from build123d import *

# Parameters (mm, degrees)
BOSS_EXTRUDE1_DEPTH = 133.35
SKETCH2_R           = 1.2
SKETCH2_R_2         = 19.75
CUT_EXTRUDE1_DEPTH  = 187.593999065
SKETCH3_W           = 133.35
SKETCH3_H           = 3.175
BOSS_EXTRUDE2_DEPTH = 3.175
FILLET1_R           = 3.175
SKETCH5_R           = 15
CUT_EXTRUDE2_DEPTH  = 189.467318942
SKETCH6_R           = 6
SKETCH6_R_2         = 5.999988
CUT_EXTRUDE3_DEPTH  = 189.467318942


with BuildPart() as part:
    # Sketch1 → Boss-Extrude1 (new body)
    with BuildSketch(Plane.XY):
        Polygon((110.49, -69.425000088), (0, 0), (0, 3.175), (110.49, -66.250000088), align=None)
    extrude(amount=BOSS_EXTRUDE1_DEPTH)

    # Sketch2 → Cut-Extrude1 (cut, through all)
    with BuildSketch(Plane(origin=(1.430283892, 2.276299128, 0), x_dir=(0.8467258159330607, -0.5320295035357462, 0), z_dir=(0.5320295035357462, 0.8467258159330607, 0))):
        with Locations(Location((26.260806326, -83.175, 0), (0, 0, 180))):
            Circle(SKETCH2_R)
        with Locations(Location((42.760806326, -66.675, 0), (0, 0, 180))):
            Circle(SKETCH2_R_2)
        with Locations(Location((59.260806326, -83.175, 0), (0, 0, 180))):
            Circle(SKETCH2_R)
        with Locations(Location((26.260806326, -50.175, 0), (0, 0, 180))):
            Circle(SKETCH2_R)
        with Locations(Location((59.260806326, -50.175, 0), (0, 0, 180))):
            Circle(SKETCH2_R)
    extrude(amount=-CUT_EXTRUDE1_DEPTH, mode=Mode.SUBTRACT)

    # Sketch3 → Boss-Extrude2 (add)
    with BuildSketch(Plane(origin=(110.49, 0, 0), x_dir=(0, 0, -1), z_dir=(1, 0, 0))):
        with Locations((-66.675, -67.837500088)):
            Rectangle(SKETCH3_W, SKETCH3_H)
    extrude(amount=BOSS_EXTRUDE2_DEPTH)

    # Fillet1
    fillet1_edges = [part.edges().sort_by_distance(p)[0] for p in [
        (113.665, -66.250000088, 66.675),
    ]]
    fillet(fillet1_edges, radius=FILLET1_R - 0.0001)  # a hair under: the kernel refuses the full size

    # Sketch5 → Cut-Extrude2 (cut, through all)
    with BuildSketch(Plane(origin=(1.430283892, 2.276299128, 0), x_dir=(0.8467258159330606, -0.5320295035357464, 0), z_dir=(0.5320295035357464, 0.8467258159330606, 0))):
        with Locations(Location((20.851690059, -111.125, 0), (0, 0, 180))):
            Circle(SKETCH5_R)
        with Locations(Location((20.851690059, -22.225, 0), (0, 0, 180))):
            Circle(SKETCH5_R)
    extrude(amount=-CUT_EXTRUDE2_DEPTH, mode=Mode.SUBTRACT)

    # Sketch6 → Cut-Extrude3 (cut, through all)
    with BuildSketch(Plane(origin=(1.430283892, 2.276299128, 0), x_dir=(0.8467258159330606, -0.5320295035357464, 0), z_dir=(0.5320295035357464, 0.8467258159330606, 0))):
        with Locations(Location((87.210806326, -46.355, 0), (0, 0, 180))):
            Circle(SKETCH6_R)
        with Locations(Location((87.210806326, -26.035, 0), (0, 0, 180))):
            Circle(SKETCH6_R)
        with Locations(Location((87.210806326, -86.995, 0), (0, 0, 180))):
            Circle(SKETCH6_R)
        with Locations(Location((87.210806326, -107.315, 0), (0, 0, 180))):
            Circle(SKETCH6_R)
        with Locations(Location((87.210806326, -66.675, 0), (0, 0, 180))):
            Circle(SKETCH6_R_2)
    extrude(amount=-CUT_EXTRUDE3_DEPTH, mode=Mode.SUBTRACT)


solid = part.part
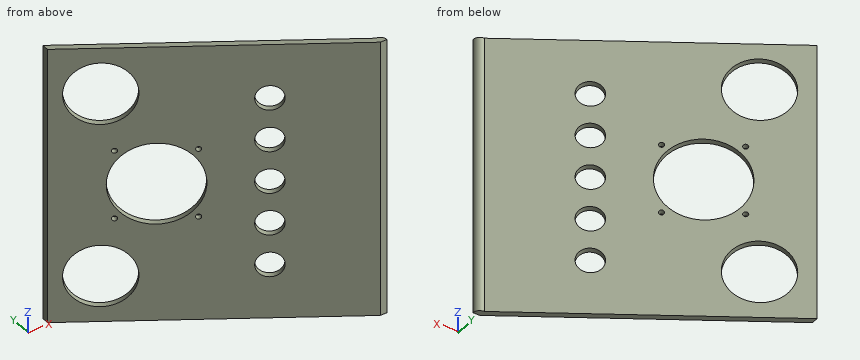
CAD build for the part. Positions are in the model's coordinates, mm. Give positions to 0.01 mm unless a question says otherwise; leave off trailing zeros. One line per question, with ' | ' between items. Start each with the question number.
1. Probe L1, parallel to Y at x = 84, z = 60; L2, parallel to Y at x = 107, z = 71; L3, parallel to X at y = -22.5, z = 11.5. List the from-to ranges inside material, lowest first. Write a range as from..to.
2. Saw through at A-A on z = 105.5. State how many separate pieces and enclosed holes the cut face has, plus the area to 3 significant figures.
3. Flat gauge pins, fed straight in: pin 1 (3 mm diameter, centred on x = 61, z = 26, fed in from +Y); pin 2 (1 mm diameter, centred on y = -39.5, z = 68, fed in from -X); pin 3 (3 mm diameter, centred on y = -50, z = 35, fed in from +X); pin 4 (8 mm diameter, centred on x = 17.5, z = 33, fed in from -Y). Where does each tip first touch, or does it go through?
Result sheet:
1) L1: y = -52.78..-49.61 | L2: y = -67.23..-64.06 | L3: x = 35.81..40.86
2) separate pieces: 3 | enclosed holes: 0 | area: 253 mm^2
3) pin 1: stops at y = -34.21 | pin 2: stops at x = 62.07 | pin 3: stops at x = 87.02 | pin 4: passes through
